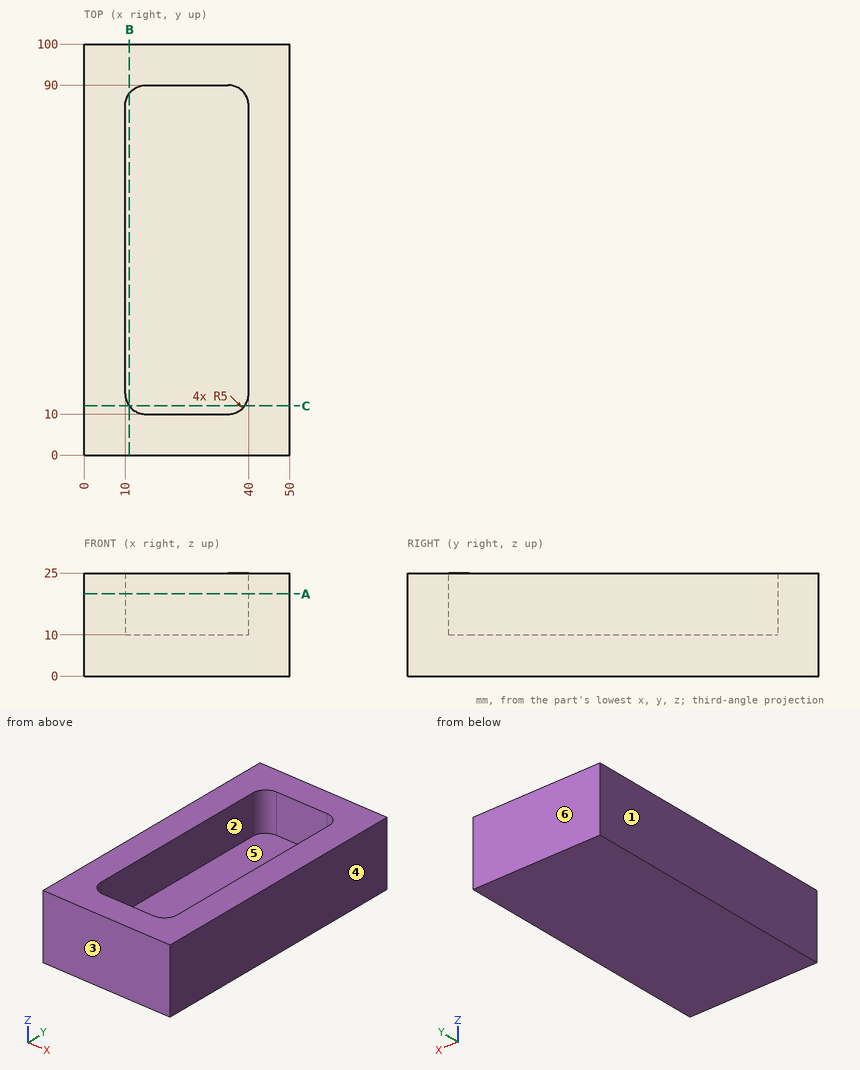
Study the drawing (mm; zero at the part's minimum x, y, z) and answer. A direction names the side the tool comes from. Coordinates: 2 decimals unless noted, no trailing zeros. Write each loop counter-clockwise with the first axis right and the second up, starting at its lowest first coordinate (ties: lowest second). Pieces come first, ordered by that corner, then holes.
Q1. This flat-tipped pin is pushed along its axis until it touches: pin 1 Ø2 at (x, y) = (27.5, 51) entering from +Z. Where does it stop, or does it pass through?
Q2. Which of the six approach directions +Z, -Z, +X, -X, +Y, -Y give full straight-line access (tool end or side, diameter ignored) to the marked faces 1 and 2?
Q3. A cutting plane is placed at B-B, the plane x = 11. Give the vertices of the cut face in (y, z), then the cut area to 3 significant figures.
Q4. A cutting plane is placed at A-A, the plane z = 20. Give the vertices of the cut face in (x, y), then the cut area to 3 significant figures.
Q5. Determine the mould class of the marked faces 3, 4, 5 and 6 for opening direction Y: released by +Y, released by -Y, zero draft, split by the parting line, or undercut.
Q6. Find the intervals of material crossed by line 1 (X direction, y = 21.5, z = 12.25); line 2 (Y direction, x = 22, z = 23.75); line 3 (Z direction, x = 33, y = 49), in increasing order.
Q7. A cutting plane is placed at C-C, the plane y = 12. Give the vertices of the cut face in (x, z), then the cut area to 3 significant figures.
Findings below:
1. pin 1: stops at z = 10
2. face 1: +Z, -Z, -X, +Y, -Y
2. face 2: +Z
3. outline: (0, 0) - (100, 0) - (100, 25) - (88, 25) - (88, 10) - (12, 10) - (12, 25) - (0, 25) - close
3. area: 1,360 mm2
4. outline: (0, 0) - (50, 0) - (50, 100) - (0, 100) - close; hole (10, 15) arc R5 ccw to (15, 10) - (35, 10) arc R5 ccw to (40, 15) - (40, 85) arc R5 ccw to (35, 90) - (15, 90) arc R5 ccw to (10, 85) - close
4. area: 2,620 mm2
5. face 3: released by -Y
5. face 4: zero draft
5. face 5: undercut
5. face 6: released by +Y
6. line 1: x = 0 to 10, 40 to 50
6. line 2: y = 0 to 10, 90 to 100
6. line 3: z = 0 to 10
7. outline: (0, 0) - (50, 0) - (50, 25) - (39, 25) - (39, 10) - (11, 10) - (11, 25) - (0, 25) - close
7. area: 830 mm2
